Autodesk Inventor part; units mm, degrees
ref_plane "YZ Plane" through (0, 0, 0) normal (1, 0, 0) x (0, 1, 0)
ref_plane "XZ Plane" through (0, 0, 0) normal (0, 1, 0) x (-1, 0, 0)
ref_plane "XY Plane" through (0, 0, 0) normal (0, 0, 1) x (1, 0, 0)
sketch "Skizze1" plane through (0, 0, 0) normal (0, 1, 0) x (-1, 0, 0)
  line L0 (0, 0) -> (23.3, 0)
  line L1 (23.3, 0) -> (23.3, 26.8)
  line L2 (23.3, 26.8) -> (0, 26.8)
  line L3 (0, 26.8) -> (0, 0)
  dimension "d0" = 23.3
  dimension "d1" = 26.8
extrude "Extrusion1" add sketch "Skizze1" along normal blind 0.4
sketch "Skizze2" plane through (0, 0, 0) normal (0, -1, 0) x (1, 0, 0)
  line L0 (0, 0) -> (-23.3, 0)
  line L1 (0, 26.8) -> (0, 0)
  line L2 (-23.3, 26.8) -> (0, 26.8)
  line L3 (-23.3, 0) -> (-23.3, 26.8)
  line L4 (-17.8, 3) -> (-5.5, 3)
  line L5 (-5.5, 3) -> (-5.5, 9.8)
  line L6 (-5.5, 9.8) -> (-17.8, 9.8)
  line L7 (-17.8, 9.8) -> (-17.8, 3)
  dimension "d4" = 3
  dimension "d5" = 17
  dimension "d6" = 5.5
  dimension "d7" = 5.5
extrude "Extrusion2" add sketch "Skizze2" along normal blind 1 contours L7 L6 L5 L4
sketch "Skizze3" plane through (0, -1, 0) normal (0, -1, 0) x (1, 0, 0)
  line L0 (-17.8, 3) -> (-5.5, 3)
  line L1 (-5.5, 3) -> (-5.5, 9.8)
  line L2 (-5.5, 9.8) -> (-17.8, 9.8)
  line L3 (-17.8, 9.8) -> (-17.8, 3)
  circle A0 centre (-11.65, 6.4) radius 2.9125
  point P0 (0, 0)
extrude "Extrusion3" cut sketch "Skizze3" against normal blind 1 contours A0
ref_plane "Work Plane1" through (-11.65, 0, 0) normal (-1, 0, 0) x (0, 0, 1)
properties part number "02_Nanoscopy_Chip"
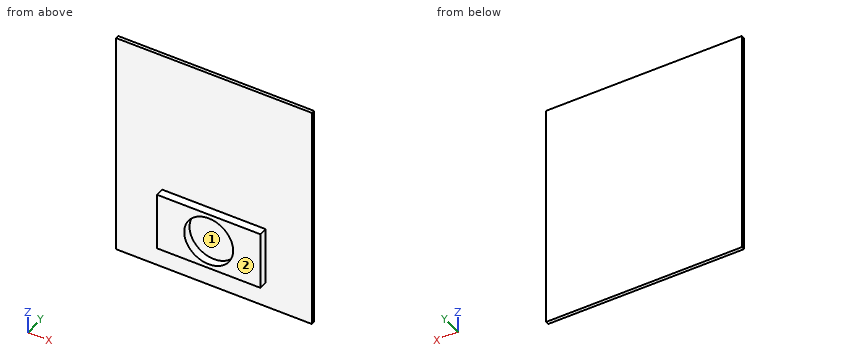
Model file for the job. Use its own axes, mm. Face numbers are marked on the shaded views. Give positions to 0.01 mm unless a question says otherwise; leave off trailing zeros. Loops run counter-clockwise (first coordinate to the right, second up) from the corner with the lowest first, then second, coordinate; pieces in that order, holes last. Notation, with made-up numbers: (45, 59) - (84, 59) arc R21 ccw to (84, 97) - close; hole circle Ø2 at (20, 52). An arc over 180 degrees is marked (long way). One line per item, written item: value. Start each with the question number.
1. Slice it at B-B (x = -11.65). List the corners of the cut face in (y, z), plus the area to 3 significant figures.
2. Probe L1, parallel to Z at x = -11.5, y = -0.15; L2, parallel to Y at x = -13.75, z = 17; L3, parallel to X at y = -0.2, z = 7.5. List the from-to ranges inside material, lowest first. Write a range as from..to.
3. Slice it at D-D (x = -6.5). List the corners of the cut face in (y, z).
4. Pin check, flat tip, straight feed: pin 1 (1 mm diameter, centred on x = -12, z = 14.5, fed in from -Y). Stop position of the tip, or through.
5. Slice it at C-C (z = 6.4). List the corners of the cut face in (x, y).
6. Pull direction Z, two halves, no side cores. Call the marked faces 1 and 2: pulls with the +Z half, pulls with the -Z half, needs draft (parallel to the pull), parting line crosses it, or undercut.
Solution:
1. outline: (-1, 3) - (0, 3) - (0, 0) - (0.4, 0) - (0.4, 26.8) - (0, 26.8) - (0, 9.8) - (-1, 9.8) - (-1, 9.31) - (0, 9.31) - (0, 3.49) - (-1, 3.49) - close
1. area: 11.7 mm^2
2. L1: z = 3..3.49, 9.31..9.8
2. L2: y = 0..0.4
2. L3: x = -17.8..-14.35, -8.95..-5.5
3. outline: (-1, 3) - (0, 3) - (0, 0) - (0.4, 0) - (0.4, 26.8) - (0, 26.8) - (0, 9.8) - (-1, 9.8) - close
4. pin 1: stops at y = 0
5. outline: (-23.3, 0) - (-17.8, 0) - (-17.8, -1) - (-14.56, -1) - (-14.56, 0) - (-8.74, 0) - (-8.74, -1) - (-5.5, -1) - (-5.5, 0) - (0, 0) - (0, 0.4) - (-23.3, 0.4) - close
6. face 1: undercut
6. face 2: needs draft
